Verification items for the finished model (mm, model axes). A direction names the side the tool comes from. Round coordinates to 2 decimals unless told otherwise and drop trailing zeros. Write each loop counter-clockwise with the first axis right and the second up, starting at its lowest first coordinate (ties: lowest second). Pieces come first, ordered by that corner, then holes. Notation, with made-up numbers: M -1.5,48.5 L 20.5,48.5 A30 ccw 20.5,76.5 Z; hole C 86,54.25 d8. An arc over 180 degrees is marked long. Write each question's results on one line, items separated by ' | '.
from build123d import *

# Parameters (mm, degrees)
SKETCH_1_R          = 55
SKETCH_1_R_2        = 41.5
EXTRUDE_1_DEPTH     = 27.6
CUT_EXTRUDE_START   = -21.6
SKETCH_2_R          = 55
SKETCH_2_R_2        = 50
CUT_EXTRUDE_1_DEPTH = 21.6
SKETCH_3_W          = 2.7
SKETCH_3_H          = 4.7
SKETCH_4_R          = 50
SKETCH_4_R_2        = 46
CUT_EXTRUDE_2_DEPTH = 2.7
SKETCH_5_R          = 1.6
CUT_EXTRUDE_3_DEPTH = 83.533387184
SKETCH_6_R          = 1.5
CUT_EXTRUDE_4_DEPTH = 6


with BuildPart() as part:
    # 草图1 → 凸台-拉伸1 (new body)
    with BuildSketch(Plane(origin=(0, 0, 0), x_dir=(1, 0, 0), z_dir=(0, 1, 0))):
        with Locations(Location((0, 0, 0), (0, 0, 90))):
            Circle(SKETCH_1_R)
        with Locations(Location((0, 0, 0), (0, 0, 90))):
            Circle(SKETCH_1_R_2, mode=Mode.SUBTRACT)
    extrude(amount=EXTRUDE_1_DEPTH)

    # 草图2 → 切除-拉伸1 (cut)
    with BuildSketch(Plane(origin=(0, 27.6, 0), x_dir=(1, 0, 0), z_dir=(0, 1, 0)).offset(CUT_EXTRUDE_START)):
        with Locations(Location((0, 0, 0), (0, 0, 90))):
            Circle(SKETCH_2_R)
        with Locations(Location((0, 0, 0), (0, 0, 270))):
            Circle(SKETCH_2_R_2, mode=Mode.SUBTRACT)
    extrude(amount=CUT_EXTRUDE_1_DEPTH, mode=Mode.SUBTRACT)

    # 草图3 → 切除-旋转1 (revolve, cut)
    with BuildSketch(Plane.XY, mode=Mode.PRIVATE) as cut_revolve_1_sk:
        with Locations((-48.65, 21.15)):
            Rectangle(SKETCH_3_W, SKETCH_3_H)
        with Locations((-48.65, 12.35)):
            Rectangle(SKETCH_3_W, SKETCH_3_H)
    revolve(cut_revolve_1_sk.sketch.rotate(Axis((0, 0, 0), (0, 1, 0)), 90), axis=Axis((0, 0, 0), (0, 1, 0)), mode=Mode.SUBTRACT)

    # 草图4 → 切除-拉伸2 (cut)
    with BuildSketch(Plane.XZ):
        with Locations(Location((0, 0, 0), (0, 0, 90))):
            Circle(SKETCH_4_R)
        with Locations(Location((0, 0, 0), (0, 0, 270))):
            Circle(SKETCH_4_R_2, mode=Mode.SUBTRACT)
    extrude(amount=-CUT_EXTRUDE_2_DEPTH, mode=Mode.SUBTRACT)

    # 草图5 → 切除-拉伸3 (cut, through all)
    with BuildSketch(Plane.XZ):
        with Locations(Location((45.612736373, 26.334525624, 0), (0, 0, 270))):
            Circle(SKETCH_5_R)
        with Locations(Location((45.612736373, -26.334525624, 0), (0, 0, 270))):
            Circle(SKETCH_5_R)
        with Locations(Location((0, -52.669051247, 0), (0, 0, 270))):
            Circle(SKETCH_5_R)
        with Locations(Location((-45.612736373, -26.334525624, 0), (0, 0, 270))):
            Circle(SKETCH_5_R)
        with Locations(Location((-45.612736373, 26.334525624, 0), (0, 0, 270))):
            Circle(SKETCH_5_R)
        with Locations(Location((0, 52.669051247, 0), (0, 0, 270))):
            Circle(SKETCH_5_R)
    extrude(amount=-CUT_EXTRUDE_3_DEPTH, mode=Mode.SUBTRACT)

    # 草图6 → 切除-拉伸4 (cut)
    with BuildSketch(Plane(origin=(0, 27.6, 0), x_dir=(1, 0, 0), z_dir=(0, 1, 0))):
        with Locations(Location((38.105117767, 22, 0), (0, 0, 270))):
            Circle(SKETCH_6_R)
        with Locations(Location((38.105117767, -22, 0), (0, 0, 270))):
            Circle(SKETCH_6_R)
        with Locations(Location((0, -44, 0), (0, 0, 270))):
            Circle(SKETCH_6_R)
        with Locations(Location((-38.105117767, -22, 0), (0, 0, 270))):
            Circle(SKETCH_6_R)
        with Locations(Location((-38.105117767, 22, 0), (0, 0, 270))):
            Circle(SKETCH_6_R)
        with Locations(Location((0, 44, 0), (0, 0, 270))):
            Circle(SKETCH_6_R)
    extrude(amount=-CUT_EXTRUDE_4_DEPTH, mode=Mode.SUBTRACT)


solid = part.part
1) Sectioned sample at C-C, the plane y = 17.5. Record the cut outline in (x, z).
Calculated:
outline: C 0,0 d100; hole C 0,0 d83
2) Depth check by flat-ended pin: P1, Ø1, axis at y = 15, z = 42.5, coming from the -X side; P2, Ø1.5, axis at x = -38.5, z = -22, coming from the +Y side; P3, Ø1.5, axis at y = 5, z = -10.5, coming from the -X side; P4, Ø1.9, axis at x = 0, z = 52.67, coming from the +Y side. Enter the tip coordinate at first touch or a pass-through.
Calculated:
P1: stops at x = -27.13 | P2: stops at y = 21.6 | P3: stops at x = -54.13 | P4: passes through
3) Access from +Z, -Z, +X, -X, +Y, -Y to the whole of each face (thin tool, end or side, straight path). Record for faces 4 (the flat face through (30, 18.8, 37)), 5 (the cylindrical face through (0.481, 2.958, -54.195)), 6 (the cylindrical face through (0.07, 24.64, -45.5)).
Calculated:
face 4: none | face 5: +Y, -Y | face 6: +Y
4) Sectioned sample at B-B, the plane x = 0. Count the separate pieces of the cut face and the enclosed holes in it, and give its area (3 significant figures).
Calculated:
separate pieces: 4 | enclosed holes: 0 | area: 382 mm²
5) Draft check along X on faces 1 (the cylindrical face through (-46.175, 12.383, -10.254)), 2 (the flat face through (38, 21.6, -22)), 3 (the flat face through (30, 10, 37)). Enter one of: pulls with the +X half, pulls with the -X half, needs draft (parallel to the pull), parting line crosses it, or undercut.
Calculated:
face 1: parting line crosses it | face 2: undercut | face 3: needs draft
6) Sectioned sample at A-A, the plane y = 26. Record the cut outline in (x, z), and give its area (3 significant figures).
Calculated:
outline: C 0,0 d100; hole C 0,0 d83; hole C -38.11,-22 d3; hole C -38.11,22 d3; hole C 0,-44 d3; hole C 0,44 d3; hole C 38.11,-22 d3; hole C 38.11,22 d3 | area: 2,400 mm²
7) Material ranges on line 1 (Y direction, x = 37, z = 30); line 2 (X direction, y = 1.85, z = 0); line 3 (Z direction, x = 37.5, y = 2), recorded low to high. Write a range as [from, to].
Calculated:
line 1: y = [2.7, 10], [14.7, 18.8], [23.5, 27.6] | line 2: x = [-55, -50], [-46, -41.5], [41.5, 46], [50, 55] | line 3: z = [-40.23, -33.07], [-26.64, -17.78], [17.78, 26.64], [33.07, 40.23]
